Autodesk Inventor part; units mm, degrees
ref_plane "Work Plane1" through (-8.2016, -3.8212, 3.81) normal (0, 0, 1) x (1, 0, 0)
ref_plane "YZ Plane" through (0, 0, 0) normal (1, 0, 0) x (0, 1, 0)
ref_plane "XZ Plane" through (0, 0, 0) normal (0, 1, 0) x (-1, 0, 0)
sketch "Sketch1" plane through (0, 0, 0) normal (0, 0, 1) x (1, 0, 0)
  line L0 (-8.8366, -0.0112) -> (13.5154, -0.0112) construction
  line L1 (-8.8366, -0.6462) -> (-2.4866, -0.6462)
  line L2 (-2.4866, -0.6462) -> (-2.4866, -1.4082)
  line L3 (-2.4866, -1.4082) -> (2.3394, -1.4082)
  line L4 (-8.8366, 1.2588) -> (13.5154, 1.2588) construction
  line L5 (-8.8366, -8.9012) -> (-7.5666, -8.9012) construction
  line L6 (2.3394, -1.4082) -> (2.3394, -3.8212)
  line L7 (4.1174, -1.4082) -> (4.1174, -3.8212)
  line L8 (4.1174, -1.4082) -> (12.4994, -1.4082)
  line L9 (12.4994, -1.4082) -> (12.4994, -0.6462)
  line L10 (12.4994, -0.6462) -> (13.5154, -0.6462)
  line L11 (13.5154, -0.6462) -> (13.5154, -0.0112)
  line L12 (-8.8366, -0.6462) -> (-8.8366, -0.0112)
  line L13 (-8.8366, -0.0112) -> (-7.5666, -0.0112)
  line L14 (-7.5666, -0.0112) -> (-7.5666, -0.3922)
  line L15 (-7.5666, -0.3922) -> (2.3394, -0.0112)
  line L16 (2.3394, -0.0112) -> (2.3394, 1.2588)
  line L17 (2.3394, 1.2588) -> (4.1174, 1.2588)
  line L18 (4.1174, -0.0112) -> (4.1174, 1.2588)
  line L19 (4.1174, -0.0112) -> (13.5154, -0.0112)
  line L20 (-8.8366, -3.8212) -> (15.1492, -3.8212) construction
  line L21 (4.1174, -7.6312) -> (4.1174, -7.6996)
  line L22 (2.3394, -3.8212) -> (4.1174, -3.8212)
  point P0 (0, 0)
  dimension "d0" = 22.352
  dimension "d4" = 0.635
  dimension "d7" = 0.762
  dimension "d11" = 1.27
  dimension "d15" = 8.382
  dimension "d17" = 0.762
  dimension "d18" = 1.27
  dimension "d19" = 0.381
  dimension "d21" = 90
  dimension "d22" = 1.016
  dimension "d23" = 9.398
  dimension "d24" = 9.398
  dimension "d25" = 11.176
  dimension "d26" = 16.002
  dimension "d27" = 1.905
  dimension "d28" = 3.175
  dimension "d29" = 8.255
  dimension "d30" = 13.5154
  dimension "d31" = 0.6462
  dimension "d32" = 1.6337
  dimension "d33" = 0
  dimension "d34" = 6.985
  dimension "d35" = 7.0534
  dimension "d36" = 22.352
  dimension "d37" = 22.352
revolve "Revolution1" add sketch "Sketch1" angle 360 about axis through (-8.8366, -3.8212, 0) along (1, 0, 0)
ref_plane "Work Plane1" through (-8.2016, -3.8212, 3.81) normal (0, 0, 1) x (1, 0, 0)
sketch "Sketch2" plane through (-8.2016, -3.8212, 3.81) normal (0, 0, 1) x (1, 0, 0)
  line L0 (-0.635, -3.81) -> (-0.635, 3.81)
  line L1 (-0.635, 0.8672) -> (4.445, 0.8672)
  line L2 (4.445, 0.8672) -> (4.445, -0.1488)
  line L3 (4.445, -0.1488) -> (-0.635, -0.1488)
  point P0 (8.2016, 3.8212)
  dimension "d44" = 5.08
  dimension "d45" = 1.016
  dimension "d46" = 2.9541
extrude "Extrusion1" cut sketch "Sketch2" against normal through all
properties part number "AHHHHHHHHHHHHHHHHHHH" material "ABS Plastic"
Part model, mm, in its own coordinate system. A direction names the side the tool comes from. Give positions to 0.01 mm unless a question says otherwise; leave off trailing zeros. Write each loop counter-clockwise with the first axis right and the second up, starting at its lowest first coordinate (ties: lowest second). Pieces come first, ordered by that corner, then holes. Notation, with made-up numbers: (52.25, -1) -> (94.25, -1) arc R19 cw to (94.25, 11) -> close; hole circle Ø10 at (-26.5, -8.75). An arc over 180 degrees is marked (long way). Put each result on its own line as item: value. Start each with the question number.
Item 1: Pin check, flat tips, straight feed: pin 1 Ø1.5 at (x, y) = (5, -6.5) entering from -Z; pin 2 Ø1.5 at (x, y) = (4, -6.5) entering from +Z; pin 3 Ø4 at (y, z) = (-4.5, 0.5) entering from -X. Stop position of each tip, or through.
Item 2: Cut at B-B (x = -6.5). List the corners of the cut face in (y, z) (3 decimals), then the cut area to 3 significant figures.
Item 3: Which spindle directions (+Z, -Z, +X, -X, +Y, -Y) get a long thin tool onto all of the face, cutting with end or side? Do faces 1 (the face through (-8.19, -7.63, 0.08)), 2 (the face through (-7.567, -0.2, 0)), 3 (the face through (8.37, -1.52, 0.72)), 4 (the face through (-0.04, -1.52, 0.72)). Say none if no direction does.
Item 4: Cut at A-A (x = 8.75). List the corners of the cut face in (y, z).
Item 5: Wall check: L1, parallel to X at y = -4.25, z = -4.25; L2, parallel to X at y = -6.5, z = -0.5; L3, parallel to Z at x = 1.5, y = -3. Give the ranges that are in metal, low to high. Write a range as [from, to].
Item 6: Pull direction Y, two halves, no side cores. Call faces 5 (the face through (13.515, -2, 3)), 6 (the face through (12.499, -1, 1)), 7 (the face through (3.241, -4.483, 5.037)): pulls with the +Y half, pulls with the -Y half, needs draft (parallel to the pull), parting line crosses it, or undercut.
Item 7: Cut at D-D (x = -1.75). List the corners of the cut face in (y, z), then the cut area to 3 significant figures.
Answer list:
1. pin 1: stops at z = -3.29
1. pin 2: stops at z = 4.7
1. pin 3: stops at x = -2.49
2. outline: (-3.97, -3.467) -> (-3.97, -3.172) arc R3.175 cw to (-3.97, 3.172) -> (-3.97, 3.467) arc R3.47 ccw to start; (-2.954, -3.36) arc R3.47 ccw to (-2.954, 3.36) -> (-2.954, 3.054) arc R3.175 cw to (-2.954, -3.054) -> close
2. area: 5.55 mm2
3. face 1: -X, -Y
3. face 2: +Y
3. face 3: +X
3. face 4: -X
4. outline: circle Ø7.62 at (-3.82, 0); hole circle Ø4.83 at (-3.82, 0)
5. L1: x = [2.34, 4.12]
5. L2: x = [-2.49, 12.5]
5. L3: z = [-3.69, -2.27], [2.27, 3.69]
6. face 5: needs draft
6. face 6: undercut
6. face 7: parting line crosses it
7. outline: circle Ø7.31 at (-3.82, 0); hole circle Ø4.83 at (-3.82, 0)
7. area: 23.6 mm2
